Here's how the part is built. I have some questions about the finished solid (model axes, mm). A direction names the side the tool comes from. Coordinates: 2 decimals unless noted, no trailing zeros. Write each loop counter-clockwise with the first axis right and the second up, starting at its lowest first coordinate (ties: lowest second). Pieces come first, ordered by that corner, then holes.
(1) Which directions (+Z, -Z, +X, -X, +Y, -Y) give clear straight access to the entire face, cutting with the end or side of a thin tool? Please do faces 1 (the flat face through (0, -23, -11)), 2 (the flat face through (-30.162, -23, 15)).
(2) Please list where these lines run through material, in increasing order: probe 1 along Z at (x, y) = (19, -20.5); probe 2 along X at (y, z) = (-41, -5).
(3) Imagine slicing it at B-B, the plane z = -10. List the corners of the cut face in (x, y) for me (1 decimal), plus the area to 3 significant figures.
(4) Imagine slicing it at C-C, the plane x = 5.5. List the corners of the cut face in (y, z) for me (3 decimals), plus the area to 3 significant figures.
(5) For pin 1 Ø6.5 at (y, z) = (-31.5, -8) entering from +X; pin 2 Ø1.5 at (x, y) = (12.5, -7.5) entering from -Z, each with a flat end and sliding along its axis, tell me the tip position at first contact or that it passes through.
(6) Thinking about a two-plate mould opening in Y: for faces 3 (the flat face through (12, -23, 50.8)), 4 (the flat face through (11, 0, 23)), 5 (the flat face through (11, -47.625, 23)), which applies, released by +Y, released by -Y, zero draft, split by the parting line, or undercut?
(7) Imagine slicing it at A-A, the plane y = -20.5. List the corners of the cut face in (x, z) for me (1 decimal), plus the area to 3 significant figures.
```python
from build123d import *

# Parameters (mm, degrees)
F0_W     = 53.975
F0_H     = 50.8
F1_DEPTH = 47.625
F2_DEPTH = 47.625


with BuildPart() as f1:
    # F0 (on Front) → F1 (new body)
    with BuildSketch(Plane.XZ):
        with Locations((26.9875, 25.4)):
            Rectangle(F0_W, F0_H)
    extrude(amount=F1_DEPTH)

    # F0 (on Front) → F2 (join, through all)
    with BuildSketch(Plane.XZ):
        Polygon((0, 50.8), (-30.1625, 50.8), (-30.1625, -22.225), (0, -22.225), (0, 0), align=None)
    extrude(amount=F2_DEPTH)


solid = f1.part
```
Recorded:
1. face 1: -Z, +X, +Y, -Y
1. face 2: +Z, -Z, -X, +Y, -Y
2. probe 1: z = 0 to 50.8
2. probe 2: x = -30.16 to 0
3. outline: (-30.2, -47.6) - (0, -47.6) - (0, 0) - (-30.2, 0) - close
3. area: 1,440 mm2
4. outline: (-47.625, 0) - (0, 0) - (0, 50.8) - (-47.625, 50.8) - close
4. area: 2,420 mm2
5. pin 1: stops at x = 0
5. pin 2: stops at z = 0
6. face 3: zero draft
6. face 4: released by +Y
6. face 5: released by -Y
7. outline: (-30.2, -22.2) - (0, -22.2) - (0, 0) - (54, 0) - (54, 50.8) - (-30.2, 50.8) - close
7. area: 4,940 mm2
